Here's how the part is built. I have some questions about the finished solid (model axes, mm). A direction names the side the tool comes from. Coordinates: 2 decimals unless noted, no trailing zeros. Write each loop counter-clockwise with the first axis right and the second up, starting at its lowest first coordinate (ties: lowest second). Pieces come first, ordered by that corner, then holes. Notation, with made-up numbers: M 2.5,11 L 58.5,11 A11 ccw 58.5,26 Z; hole C -35,31 d1. An arc over 180 degrees is marked long. Use a Markdown table: item, result.
```python
from build123d import *

# Parameters (mm, degrees)
SKETCH_1_R          = 15.5
EXTRUDE_1_DEPTH     = 17.8
CUT_EXTRUDE_START   = -6
CUT_EXTRUDE_1_DEPTH = 6


with BuildPart() as part:
    # 草图1 → 凸台-拉伸1 (new body)
    with BuildSketch(Plane(origin=(0, 0, 0), x_dir=(1, 0, 0), z_dir=(0, 1, 0))):
        with Locations(Location((0, 0, 0), (0, 0, 270))):
            Circle(SKETCH_1_R)
    extrude(amount=EXTRUDE_1_DEPTH)

    # 草图2 → 切除-拉伸1 (cut)
    with BuildSketch(Plane(origin=(0, 17.8, 0), x_dir=(1, 0, 0), z_dir=(0, 1, 0)).offset(CUT_EXTRUDE_START)):
        with BuildLine():
            Line((-7.5, 13.564659966), (-7.5, -13.564659966))
            ThreePointArc((-7.5, -13.564659966), (0, -15.5), (7.5, -13.564659966))
            Line((7.5, -13.564659966), (7.5, 13.564659966))
            ThreePointArc((7.5, 13.564659966), (0, 15.5), (-7.5, 13.564659966))
        make_face()
    extrude(amount=CUT_EXTRUDE_1_DEPTH, mode=Mode.SUBTRACT)


solid = part.part
```
1. Will these pins go through, and if not, where does the flat tip stop? pin 1 Ø7.5 at (x, z) = (1, 5.5) entering from +Y; pin 2 Ø10 at (x, y) = (-6, 5.5) entering from +Z; pin 3 Ø4 at (y, z) = (12, -4.5) entering from -X.
Answers follow:
| item | result |
|---|---|
| pin 1 | stops at y = 11.8 |
| pin 2 | stops at z = 15.47 |
| pin 3 | stops at x = -15.3 |
2. Suppose I cut it at A-A on y = 14. Write out the boundary of the cut face in (x, z), and give its area (3 significant figures).
Answers follow:
| item | result |
|---|---|
| outline | M -7.5,-13.56 L -7.5,13.56 A15.5 ccw Z; M 7.5,-13.56 A15.5 ccw 7.5,13.56 Z |
| area | 309 mm2 |
3. Suppose I cut it at B-B on z = 4.5. Write out the boundary of the cut face in (x, y).
Answers follow:
| item | result |
|---|---|
| outline | M -14.83,0 L 14.83,0 L 14.83,17.8 L 7.5,17.8 L 7.5,11.8 L -7.5,11.8 L -7.5,17.8 L -14.83,17.8 Z |
4. Suppose I cut it at C-C on y = 11. Write out the boundary of the cut face in (x, z), and give its area (3 significant figures).
Answers follow:
| item | result |
|---|---|
| outline | C 0,0 d31 |
| area | 755 mm2 |
5. Suppose I cut it at D-D on x = 0. Write out the boundary of the cut face in (y, z), and give its area (3 significant figures).
Answers follow:
| item | result |
|---|---|
| outline | M 0,-15.5 L 11.8,-15.5 L 11.8,15.5 L 0,15.5 Z |
| area | 366 mm2 |
6. Which directions (+Z, -Z, +X, -X, +Y, -Y) give clear straight access to the entire face, cutting with the end or side of a thin tool? Please do faces 1 (the face through (-7.5, 15, 0)), 2 (the face through (0, 0, 0)).
Answers follow:
| item | result |
|---|---|
| face 1 | +Z, -Z, +Y |
| face 2 | +Z, -Z, +X, -X, -Y |
7. We'd pull the mould along X, two halves only. Please class faces 3 (the face through (0.682, 8.775, -15.485)), 4 (the face through (11, 17.8, 0)), 5 (the face through (7.5, 15, 0)): +X half, -X half, draft (parallel to the pull), parting line (faces both ways), or undercut.
Answers follow:
| item | result |
|---|---|
| face 3 | parting line |
| face 4 | draft |
| face 5 | undercut |
8. I need wall thicknesses on probe 1 along X at (y, z) = (16.5, 0); probe 2 along X at (y, z) = (6, 0); probe 3 along Z at (x, y) = (7.5, 7.25). Which ranges of each line are inside material? Lowest first, please.
Answers follow:
| item | result |
|---|---|
| probe 1 | x = -15.5 to -7.5, 7.5 to 15.5 |
| probe 2 | x = -15.5 to 15.5 |
| probe 3 | z = -13.56 to 13.56 |
